Autodesk Inventor part; units mm, degrees
ref_plane "YZ Plane" through (0, 0, 0) normal (1, 0, 0) x (0, 1, 0)
ref_plane "XZ Plane" through (0, 0, 0) normal (0, 1, 0) x (-1, 0, 0)
ref_plane "XY Plane" through (0, 0, 0) normal (0, 0, 1) x (1, 0, 0)
sketch "Sketch1" plane through (0, 0, 0) normal (0, 1, 0) x (-1, 0, 0)
  line L0 (0, 0) -> (88.9, 0)
  line L1 (88.9, 0) -> (88.9, -88.9)
  line L2 (88.9, -88.9) -> (0, -88.9)
  line L3 (0, -88.9) -> (0, 0)
  line L4 (82.931, -5.969) -> (5.969, -5.969)
  line L5 (5.969, -5.969) -> (5.969, -82.931)
  line L6 (5.969, -82.931) -> (82.931, -82.931)
  line L7 (82.931, -82.931) -> (82.931, -5.969)
  point P0 (44.45, -5.969)
  dimension "d0" = 88.9
  dimension "d1" = 88.9
  dimension "d2" = 5.969
  dimension "d3" = 5.969
  dimension "d4" = 5.969
  dimension "d5" = 5.969
extrude "Extrusion1" add sketch "Sketch1" along normal blind 0.889
sketch "Sketch2" plane through (0, 0.889, 0) normal (0, 1, 0) x (1, 0, 0)
  circle A0 centre (-85.9155, 44.45) radius 1.5875
  line L0 (-88.9, 88.9) -> (-88.9, 0)
  line L1 (0, 88.9) -> (-88.9, 88.9)
  circle A1 centre (-2.9845, 44.45) radius 1.5875
  line L2 (-5.969, 82.931) -> (-5.969, 5.969)
  circle A2 centre (-44.45, 2.9845) radius 1.5875
  line L3 (-5.969, 5.969) -> (-82.931, 5.969)
  circle A3 centre (-44.45, 85.9155) radius 1.5875
  line L4 (-82.931, 82.931) -> (-5.969, 82.931)
  point P0 (0, 0)
  dimension "d8" = 3.175
  dimension "d9" = 2.9845
  dimension "d10" = 44.45
  dimension "d11" = 3.175
  dimension "d12" = 2.9845
  dimension "d13" = 3.175
  dimension "d14" = 2.9845
  dimension "d15" = 3.175
  dimension "d16" = 2.9845
extrude "Extrusion2" cut sketch "Sketch2" against normal through all
properties part number "top plate"
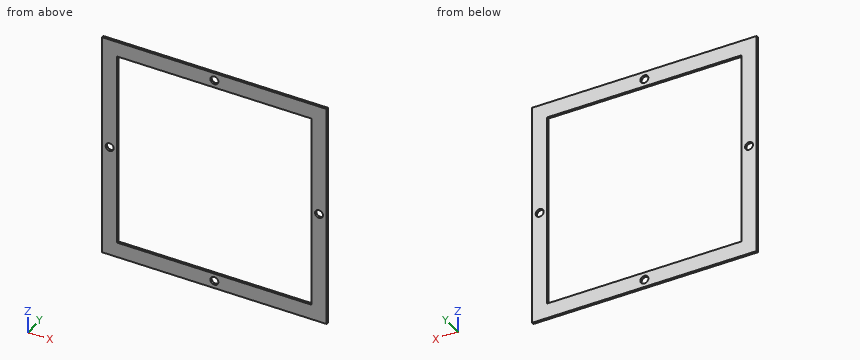
CAD build for the part. Positions are in the model's coordinates, mm. Give positions to 0.01 mm unless a question says otherwise; leave off trailing zeros. Loops run counter-clockwise (first coordinate to the right, second up) from the corner with the lowest first, then second, coordinate; pieces in that order, holes last. Notation, with made-up numbers: (54.5, -37.75) - (104.5, -37.75) arc R23 cw to (104.5, -18.75) - close; hole circle Ø4 at (46, -20). An arc over 180 degrees is marked (long way). Put each result on its own line as item: value.
Q1. Slice it at A-A (x = -65.5). Give the cut face in (y, z).
Filled in:
outline: (0, -88.9) - (0.89, -88.9) - (0.89, -82.93) - (0, -82.93) - close; (0, -5.97) - (0.89, -5.97) - (0.89, 0) - (0, 0) - close
Q2. Slice it at D-D (z = -15). Give the cut face in (x, y).
Filled in:
outline: (-88.9, 0) - (-82.93, 0) - (-82.93, 0.89) - (-88.9, 0.89) - close; (-5.97, 0) - (0, 0) - (0, 0.89) - (-5.97, 0.89) - close
Q3. Probe line 1 along Z through (x, y) = (-44.45, 0.3); line 2 along X through (y, z) = (0.65, -65). List the from-to ranges inside material, lowest first.
Filled in:
line 1: z = -88.9 to -87.5, -84.33 to -82.93, -5.97 to -4.57, -1.4 to 0
line 2: x = -88.9 to -82.93, -5.97 to 0
Q4. Slice it at B-B (z = -44.45). Give the cut face in (x, y), plus the area to 3 significant figures.
Filled in:
outline: (-88.9, 0) - (-87.5, 0) - (-87.5, 0.89) - (-88.9, 0.89) - close; (-84.33, 0) - (-82.93, 0) - (-82.93, 0.89) - (-84.33, 0.89) - close; (-5.97, 0) - (-4.57, 0) - (-4.57, 0.89) - (-5.97, 0.89) - close; (-1.4, 0) - (0, 0) - (0, 0.89) - (-1.4, 0.89) - close
area: 4.97 mm²
Q5. Flat gauge pin, fed straight in: pin 1 (5 mm diameter, centred on x = -44.45, z = -2.98, fed in from +Y). Where does the tip first touch, or does it go through?
Filled in:
pin 1: stops at y = 0.89
Q6. Slice it at C-C (x = -44.45). Give the cut face in (y, z), plus the area to 3 significant figures.
Filled in:
outline: (0, -88.9) - (0.89, -88.9) - (0.89, -87.5) - (0, -87.5) - close; (0, -84.33) - (0.89, -84.33) - (0.89, -82.93) - (0, -82.93) - close; (0, -5.97) - (0.89, -5.97) - (0.89, -4.57) - (0, -4.57) - close; (0, -1.4) - (0.89, -1.4) - (0.89, 0) - (0, 0) - close
area: 4.97 mm²
